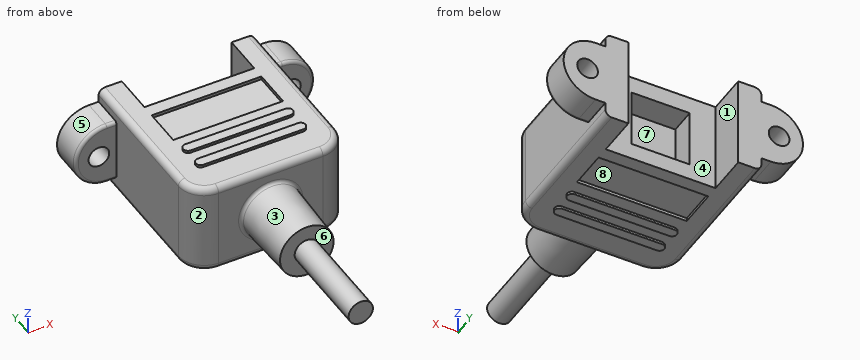
Autodesk Inventor part; units mm, degrees
ref_plane "Work Plane1" through (12.075, 8.075, 7.1) normal (0, 0, -1) x (-1, 0, 0)
ref_plane "YZ Plane" through (0, 0, 0) normal (1, 0, 0) x (0, 1, 0)
ref_plane "XZ Plane" through (0, 0, 0) normal (0, 1, 0) x (-1, 0, 0)
sketch "Sketch1" plane through (0, 0, 0) normal (0, 0, 1) x (1, 0, 0)
  line L0 (8.075, -13.075) -> (-8.075, -13.075)
  line L1 (-12.075, -9.075) -> (-12.075, 13.075)
  line L2 (-12.075, 13.075) -> (12.075, 13.075)
  line L3 (12.075, 13.075) -> (12.075, -9.075)
  line L4 (12.075, -13.075) -> (-12.075, 13.075) construction
  line L5 (-12.075, -13.075) -> (12.075, 13.075) construction
  arc A0 (-12.075, -9.075) -> (-8.075, -13.075) centre (-8.075, -9.075) ccw
  arc A1 (8.075, -13.075) -> (12.075, -9.075) centre (8.075, -9.075) ccw
  point P0 (0, 0)
  dimension "d0" = 24.15
  dimension "d1" = 26.15
  dimension "d2" = 4
extrude "Extrusion1" add sketch "Sketch1" along normal blind 14.2
sketch "Sketch2" plane through (-12.075, 13.075, 0) normal (0, 1, 0) x (1, 0, 0)
  line L0 (24.15, 0) -> (24.15, -14.2) construction
  line L1 (24.15, 0) -> (0, 0) construction
  line L2 (4, -14.2) -> (20.15, -14.2) construction
  line L3 (12.075, -14.2) -> (12.075, 8.7449) construction
  arc A0 (25.65, -12.05) -> (25.65, -2.15) centre (25.65, -7.1) ccw
  line L4 (24.15, 0) -> (24.15, -14.2) construction
  line L5 (24.15, -7.1) -> (-4.8998, -7.1) construction
  line L6 (30.6, -19.6482) -> (30.6, 9.5146) construction
  line L7 (25.65, -2.15) -> (24.15, -2.15)
  line L8 (25.65, -12.05) -> (24.15, -12.05)
  line L9 (24.15, -2.15) -> (24.15, -12.05)
  point P0 (12.075, 0)
  dimension "d5" = 9.9
  dimension "d6" = 6.45
extrude "Extrusion2" add sketch "Sketch2" against normal blind 5
sketch "Sketch3" plane through (-12.075, 8.075, 0) normal (0, -1, 0) x (1, 0, 0)
  line L0 (24.15, 8.6877) -> (26.9, 10.2754) construction
  line L1 (26.9, 10.2754) -> (29.65, 8.6877) construction
  line L2 (29.65, 8.6877) -> (29.65, 5.5123) construction
  line L3 (29.65, 5.5123) -> (26.9, 3.9246) construction
  line L4 (26.9, 3.9246) -> (24.15, 5.5123) construction
  line L5 (24.15, 5.5123) -> (24.15, 8.6877) construction
  line L6 (24.15, 2.15) -> (24.15, 12.05) construction
  arc A0 (25.65, 2.15) -> (25.65, 12.05) centre (25.65, 7.1) ccw construction
  line L7 (25.65, 7.1) -> (35.3892, 7.1) construction
  line L8 (26.9, 10.2754) -> (26.9, 3.9246) construction
  point P0 (12.075, 0)
  point P1 (26.9, 7.1)
  point P2 (26.9, 7.1)
  dimension "d9" = 5.5
sketch "Sketch4" plane through (-12.075, 8.075, 0) normal (0, -1, 0) x (1, 0, 0)
  circle A0 centre (26.9, 7.1) radius 1.6
  point P0 (12.075, 0)
  dimension "d10" = 3.2
extrude "Extrusion3" cut sketch "Sketch4" against normal blind 5
mirror "Mirror1" about plane through (0, 0, 0) normal (1, 0, 0) of "Extrusion2", "Extrusion3"
sketch "Sketch5" plane through (-12.075, 13.075, 0) normal (0, 1, 0) x (1, 0, 0)
  line L0 (24.15, 0) -> (0, 0) construction
  line L1 (0, 0) -> (0, -2.15) construction
  line L2 (24.15, -14.2) -> (0, -14.2)
  line L3 (20.575, 0) -> (3.575, 0)
  line L4 (3.575, 0) -> (3.575, -14.2)
  line L5 (3.575, -14.2) -> (20.575, -14.2)
  line L6 (20.575, -14.2) -> (20.575, 0)
  line L7 (12.075, 0) -> (12.075, -22.6768) construction
  dimension "d13" = 17
extrude "Extrusion4" cut sketch "Sketch5" against normal blind 6.3
sketch "Sketch6" plane through (-8.075, -13.075, 0) normal (0, -1, 0) x (1, 0, 0)
  circle A0 centre (8.075, 7.1) radius 4.5
  line L0 (0, 0) -> (16.15, 0) construction
  line L1 (20.15, 0) -> (20.15, 14.2) construction
  point P0 (8.075, 0)
  dimension "d16" = 9
  dimension "d17" = 7.1
  dimension "d18" = 12.075
extrude "Extrusion5" add sketch "Sketch6" along normal blind 10 draft -2
sketch "Sketch7" plane through (0, -23.075, 7.1) normal (0, -1, 0) x (1, 0, 0)
  circle A0 centre (0, 0) radius 4.1508
  circle A1 centre (0, 0) radius 1.88
  point P0 (0, -7.1)
  dimension "d21" = 3.76
extrude "Extrusion6" add sketch "Sketch7" along normal blind 15 contours A1
sketch "Sketch8" plane through (-12.075, 6.775, 0) normal (0, 1, 0) x (1, 0, 0)
  line L0 (3.575, -14.2) -> (3.575, 0) construction
  line L1 (3.575, 0) -> (20.575, 0) construction
  circle A0 centre (12.075, -7.1) radius 1.88 construction
  line L2 (18.135, -12.625) -> (6.015, -12.625)
  line L3 (6.015, -12.625) -> (6.015, -1.575)
  line L4 (6.015, -1.575) -> (18.135, -1.575)
  line L5 (18.135, -1.575) -> (18.135, -12.625)
  line L6 (18.135, -12.625) -> (6.015, -1.575) construction
  line L7 (6.015, -12.625) -> (18.135, -1.575) construction
  point P0 (12.075, 0)
  dimension "d24" = 12.12
  dimension "d25" = 11.05
fillet "Fillet1" radius 1 10 edges at (-10.9034, -11.9034, 0) (0, -13.075, 0) (10.9034, -11.9034, 0) (12.075, 2, 0) (-12.075, 2, 0) (-10.9034, -11.9034, 14.2) (0, -13.075, 14.2) (10.9034, -11.9034, 14.2) (12.075, 2, 14.2) (-12.075, 2, 14.2)
sketch "Sketch9" plane through (0, 0, 0) normal (0, 0, -1) x (-1, 0, 0)
  line L0 (0, -48.305) -> (0, 23.305) construction
  line L1 (8.5, 4.775) -> (-8.5, 4.775)
  line L2 (-8.5, 4.775) -> (-8.5, -1.225)
  line L3 (-8.5, -1.225) -> (8.5, -1.225)
  line L4 (8.5, -1.225) -> (8.5, 4.775)
  line L5 (8.5, 4.775) -> (-8.5, -1.225) construction
  line L6 (-8.5, 4.775) -> (8.5, -1.225) construction
  line L7 (-8.5, 6.775) -> (8.5, 6.775)
  point P0 (0, 0)
  point P1 (0, 1.775)
  dimension "d27" = 17
  dimension "d28" = 6
  dimension "d29" = 2
extrude "Extrusion7" cut sketch "Sketch9" against normal blind 0.5
sketch "Sketch10" plane through (0, 0, 0) normal (0, 0, -1) x (-1, 0, 0)
  line L0 (8.5, -1.225) -> (-8.5, -1.225) construction
  line L1 (0, -48.305) -> (0, 23.305) construction
  line L2 (-7.75, -3.225) -> (7.75, -3.225)
  line L3 (8.5, -3.975) -> (8.5, -3.975)
  line L4 (7.75, -4.725) -> (-7.75, -4.725)
  line L5 (-8.5, -3.975) -> (-8.5, -3.975)
  line L6 (-8.5, -3.225) -> (8.5, -4.725) construction
  line L7 (8.5, -3.225) -> (-8.5, -4.725) construction
  line L8 (-7.75, -6.725) -> (7.75, -6.725)
  line L9 (8.5, -7.475) -> (8.5, -7.475)
  line L10 (7.75, -8.225) -> (-7.75, -8.225)
  line L11 (-8.5, -7.475) -> (-8.5, -7.475)
  line L12 (-8.5, -6.725) -> (8.5, -8.225) construction
  line L13 (8.5, -6.725) -> (-8.5, -8.225) construction
  arc A0 (7.75, -8.225) -> (8.5, -7.475) centre (7.75, -7.475) ccw
  arc A1 (8.5, -7.475) -> (7.75, -6.725) centre (7.75, -7.475) ccw
  arc A2 (-8.5, -7.475) -> (-7.75, -8.225) centre (-7.75, -7.475) ccw
  arc A3 (-7.75, -6.725) -> (-8.5, -7.475) centre (-7.75, -7.475) ccw
  arc A4 (-8.5, -3.975) -> (-7.75, -4.725) centre (-7.75, -3.975) ccw
  arc A5 (-7.75, -3.225) -> (-8.5, -3.975) centre (-7.75, -3.975) ccw
  arc A6 (8.5, -3.975) -> (7.75, -3.225) centre (7.75, -3.975) ccw
  arc A7 (7.75, -4.725) -> (8.5, -3.975) centre (7.75, -3.975) ccw
  point P0 (0, 0)
  point P1 (0, -3.975)
  point P2 (0, -7.475)
  dimension "d32" = 17
  dimension "d33" = 1.5
  dimension "d34" = 2
  dimension "d35" = 17
  dimension "d36" = 1.5
  dimension "d37" = 2
  dimension "d38" = 0.75
extrude "Extrusion8" add sketch "Sketch10" along normal blind 0.4
ref_plane "Work Plane1" through (12.075, 8.075, 7.1) normal (0, 0, -1) x (-1, 0, 0)
mirror "Mirror2" about plane through (12.075, 8.075, 7.1) normal (0, 0, -1) of "Extrusion7", "Extrusion8"
fillet "Fillet2" radius 0.5 1 edges at (-4.5, -13.075, 7.1)
fillet "Fillet3" radius 0.5 6 edges at (-12.825, 8.075, 12.05) (-12.825, 8.075, 2.15) (-18.525, 8.075, 7.1) (12.825, 8.075, 12.05) (12.825, 8.075, 2.15) (18.525, 8.075, 7.1)
sketch "Sketch11" plane through (-12.075, 6.775, 0) normal (0, 1, 0) x (1, 0, 0)
  line L0 (7.575, -2.5467) -> (16.575, -2.5467)
  line L1 (16.575, -2.5467) -> (16.575, -11.5467)
  line L2 (16.575, -11.5467) -> (7.575, -11.5467)
  line L3 (7.575, -11.5467) -> (7.575, -2.5467)
  line L4 (7.575, -2.5467) -> (16.575, -11.5467) construction
  line L5 (16.575, -2.5467) -> (7.575, -11.5467) construction
  point P0 (12.075, 0)
  point P1 (12.075, -7.0467)
  dimension "d43" = 9
  dimension "d44" = 9
extrude "Extrusion9" cut sketch "Sketch11" against normal blind 4
properties part number "USB Cable B Male to B Female 90 degrees" material "Nylon 6/6"
For this review, take the finished solid that the model builds, in its own axes (mm). Face numbers are marked on the shaded views. A direction names the side the tool comes from. Round coordinates to 2 decimals unless told otherwise and drop trailing zeros. Write each loop counter-clockwise with the first axis right and the second up, starting at its lowest first coordinate (ties: lowest second). Pieces come first, ordered by that corner, then holes. Notation, with made-up numbers: (51.5, 40) -> (96.5, 40) arc R18 ccw to (96.5, 73) -> close; hole circle Ø8 at (-23.75, 77). An arc over 180 degrees is marked (long way). Use CSV: the item, a comma, the result in double quotes.
(1) Consider section B-B, the plane z = 7.1. Give the number of separate pieces and of enclosed holes in the cut face, plus the area to 3 significant figures.
Computed values:
separate pieces,"3"
enclosed holes,"0"
area,"657 mm²"
(2) To check wall thickness, follow L1, parallel to X at y = 8, z = 5.5 (3 decimals); L2, parallel to X at y = 9.5, z = 6.25; L3, parallel to Y at x = -15, z = 8.75 (3 decimals). State the ranges of each line that lie inside material, in increasing order. Write a range as [from, to].
Computed values:
L1,"[-12.075, -8.5], [8.5, 12.075]"
L2,"[-18.45, -16.18], [-13.47, -8.5], [8.5, 13.47], [16.18, 18.45]"
L3,"[8.075, 13.075]"
(3) For the marked faces 4, 5, 6, 7 and 8, list the 3-axis set-ups (+Z, -Z, +X, -X, +Y, -Y) from which the entire face can be reached by the end or side of a thin tool; tool diameter is ignored.
Computed values:
face 4,"+Z, -Z, +Y"
face 5,"-X, +Y, -Y"
face 6,"-Y"
face 7,"+Y"
face 8,"-Z"
(4) Consider section C-C, the plane y = -18.5. Give the boundary of the cut face in (x, z).
Computed values:
outline,"circle Ø8.62 at (0, 7.1)"
(5) Draft analysis for pull direction X (two halves, no side actions). For the marked faces 1, 2 and 3, state which applies: +X half, -X half, draft (parallel to the pull), parting line (faces both ways), or undercut.
Computed values:
face 1,"undercut"
face 2,"-X half"
face 3,"parting line"
(6) Clearance check with flat-ended pins moving along their axes: P1, Ø3, axis at x = 4, y = -19.5, coming from the +Z side; P2, Ø3, axis at x = 1, y = 5.5, coming from the +Z side; P3, Ø0.6, axis at y = 1.5, z = 0.5, coming from the -X side. State where each tip first meets the part, or that it passes through.
Computed values:
P1,"z = 10.57"
P2,"z = 14.2"
P3,"x = -12.05"
